Source: CAD feature listing. Evaluate the final solid. Frame: model axes, mm. A direction names the side the tool comes from. Round coordinates to 2 decimals unless told otherwise and drop trailing zeros. Order: outer loops, then holes, each group sorted by start corner. A loop starts at its lowest first (then second) coordinate and runs counter-clockwise, first axis right, second up. Notation, with made-up numbers: (79.25, 20) - (103.25, 20) arc R29 ccw to (103.25, 52) - close; hole circle Ø3 at (79, -39.75). An arc over 180 degrees is marked (long way). Put each result on its own line as item: value. Start each with the question number.
1) Section C-C on z = 39.5. Output: boundary loops of the cut face in (x, y), then the cut area to 3 significant figures.
2) Section D-D on y = 13. State how many separate pieces and enclosed holes the cut face has, then the cut area to 3 significant figures.
3) Mould query, pull axis Z, two halves, no side actions, for faces 1 (the face through (-17, 3, 30)), 2 (the face through (-23, 8, -15.011)), 3 (the face through (7, 16, 29)), 4 (the face through (-52.111, 9.409, 60.233)). Classes: +Z half, -Z half, draft (parallel to the pull), parting line (faces both ways), or undercut.
4) Section A-A on x = -7. Output: boundary loops of the cut face in (y, z).
5) Section B-B on z = 29. Output: boundary loops of the cut face in (x, y), then the cut area to 3 significant figures.
6) Line query: probe 1 along X at (y, z) = (14.5, 50); probe 2 along Z at (x, y) = (-12.5, 8.75); probe 3 along X at (y, z) = (11.25, 65.5). Output: solid intervals per line, ascending. Write a range as [from, to].
7) Contact query for flat-ended pins moving along their axis: P1, Ø1, axis at y = 8.5, z = 35, coming from the -X side; P2, Ø14.5, axis at x = -33.5, z = 29, coming from the +Y side; P3, Ø1.5, axis at x = -51, z = 66.5, coming from the +Y side. Output: stop coordinate, or through.
8) Access query for faces 5 (the face through (-57, 4, 20.989)), 6 (the face through (3.67, 10.93, 67.62)), 7 (the face through (-58.032, 11, 29)). Directions: +Z, -Z, +X, -X, +Y, -Y. A direction counts if a zero-diameter tool reaches every point of the face in a straight line with its end or side. Return the directions, or none.
Autodesk Inventor part; units mm, degrees
ref_plane "YZ Plane" through (0, 0, 0) normal (1, 0, 0) x (0, 1, 0)
ref_plane "XZ Plane" through (0, 0, 0) normal (0, 1, 0) x (-1, 0, 0)
ref_plane "XY Plane" through (0, 0, 0) normal (0, 0, 1) x (1, 0, 0)
sketch "Sketch1" plane through (0, 0, 0) normal (0, 1, 0) x (-1, 0, 0)
  line L0 (58.0321, 73.1889) -> (-11.1179, 73.1889)
  line L1 (-11.1179, 73.1889) -> (-11.1179, -15.0111)
  line L2 (-11.1179, -15.0111) -> (58.0321, -15.0111)
  line L3 (58.0321, -15.0111) -> (58.0321, 73.1889)
  point P0 (0, 0)
  dimension "d0" = 88.2
  dimension "d1" = 69.15
extrude "Extrusion1" add sketch "Sketch1" along normal blind 3
sketch "Sketch2" plane through (0, 3, 0) normal (0, 1, 0) x (1, 0, 0)
  line L0 (-58.0321, -73.1889) -> (11.1179, -73.1889)
  line L1 (11.1179, -73.1889) -> (11.1179, 15.0111)
  line L2 (-58.0321, -73.1889) -> (11.1179, -73.1889)
  line L3 (11.1179, -73.1889) -> (11.1179, 15.0111)
  line L4 (11.1179, 15.0111) -> (-58.0321, 15.0111)
  line L5 (-58.0321, 15.0111) -> (-58.0321, -73.1889)
  line L6 (-53.0321, -68.1889) -> (6.1179, -68.1889)
  line L7 (6.1179, -68.1889) -> (6.1179, 10.0111)
  line L8 (6.1179, 10.0111) -> (-53.0321, 10.0111)
  line L9 (-53.0321, 10.0111) -> (-53.0321, -68.1889)
  line L10 (-58.0321, 15.0111) -> (-58.0321, -73.1889)
  line L11 (-58.0321, -73.1889) -> (-47.0321, -73.1889)
  line L12 (-47.0321, -73.1889) -> (-47.0321, -62.1889)
  line L13 (-47.0321, -62.1889) -> (-58.0321, -62.1889)
  line L14 (-58.0321, -62.1889) -> (-58.0321, -73.1889)
  line L15 (-58.0321, 15.0111) -> (-47.0321, 15.0111)
  line L16 (-47.0321, 15.0111) -> (-47.0321, 4.0111)
  line L17 (-47.0321, 4.0111) -> (-58.0321, 4.0111)
  line L18 (-58.0321, 4.0111) -> (-58.0321, 15.0111)
  line L19 (11.1179, 15.0111) -> (0.1179, 15.0111)
  line L20 (0.1179, 15.0111) -> (0.1179, 4.0111)
  line L21 (0.1179, 4.0111) -> (11.1179, 4.0111)
  line L22 (11.1179, 4.0111) -> (11.1179, 15.0111)
  line L23 (11.1179, -73.1889) -> (0.1179, -73.1889)
  line L24 (0.1179, -73.1889) -> (0.1179, -62.1889)
  line L25 (0.1179, -62.1889) -> (11.1179, -62.1889)
  line L26 (11.1179, -62.1889) -> (11.1179, -73.1889)
  arc A0 (1.3427, -62.1889) -> (6.1179, -57.4137) centre (1.3427, -57.4137) ccw
  arc A1 (-4.6573, -68.1889) -> (0.1179, -63.4137) centre (-4.6573, -63.4137) ccw
  arc A2 (-47.0321, -63.4137) -> (-42.2569, -68.1889) centre (-42.2569, -63.4137) ccw
  arc A3 (-53.0321, -57.4137) -> (-48.2569, -62.1889) centre (-48.2569, -57.4137) ccw
  arc A4 (-48.2569, 4.0111) -> (-53.0321, -0.7641) centre (-48.2569, -0.7641) ccw
  arc A5 (-42.2569, 10.0111) -> (-47.0321, 5.2359) centre (-42.2569, 5.2359) ccw
  arc A6 (0.1179, 5.2359) -> (-4.6573, 10.0111) centre (-4.6573, 5.2359) ccw
  arc A7 (6.1179, -0.7641) -> (1.3427, 4.0111) centre (1.3427, -0.7641) ccw
  point P0 (0, 0)
  dimension "d4" = 5
  dimension "d5" = 5
  dimension "d6" = 5
  dimension "d7" = 5
  dimension "d8" = 6
  dimension "d9" = 6
  dimension "d10" = 6
  dimension "d11" = 6
  dimension "d12" = 6
  dimension "d13" = 6
  dimension "d14" = 6
  dimension "d15" = 6
  dimension "d16" = 4.7752
  dimension "d17" = 4.7752
  dimension "d18" = 4.7752
  dimension "d19" = 4.7752
  dimension "d20" = 4.7752
  dimension "d21" = 4.7752
  dimension "d22" = 4.7752
  dimension "d23" = 4.7752
  dimension "d24" = 4.7752
  dimension "d25" = 4.7752
  dimension "d26" = 4.7752
  dimension "d27" = 4.7752
  dimension "d28" = 4.7752
  dimension "d29" = 4.7752
  dimension "d30" = 4.7752
  dimension "d31" = 4.7752
  dimension "d32" = 4.7752
  dimension "d33" = 4.7752
  dimension "d34" = 4.7752
  dimension "d35" = 4.7752
  dimension "d36" = 4.7752
  dimension "d37" = 4.7752
  dimension "d38" = 4.7752
  dimension "d39" = 4.7752
extrude "Extrusion3" add sketch "Sketch2" along normal blind 13 contours L5 L13 L9 L6 L12 L0 | L12 L6 L24 L0 | L5 L17 L9 L13 | L24 L6 L7 L25 L1 L0 | L12 A2 L6 | L6 L9 L13 L12 | L5 L4 L16 L8 L9 L17 | L9 A3 L13 | L24 L25 L7 L6 | L6 A1 L24 | L17 A4 L9 | L9 L8 L16 L17 | L25 L7 L21 L1 | L4 L20 L8 L16 | L21 L7 L8 L20 L4 L1 | L25 A0 L7 | L8 A5 L16 | L21 L20 L8 L7 | L7 A7 L21 | L20 A6 L8
fillet "Fillet1" radius 4.7752 4 edges at (0.1179, 9.5, 62.1889) (-47.0321, 9.5, 62.1889) (-47.0321, 9.5, -4.0111) (0.1179, 9.5, -4.0111)
fillet "Fillet2" radius 10 4 edges at (11.1179, 8, 73.1889) (-58.0321, 8, 73.1889) (11.1179, 8, -15.0111) (-58.0321, 8, -15.0111)
sketch "Sketch4" plane through (11.1179, 0, 63.1889) normal (1, 0, 0) x (0, 0, -1)
  point P0 (63.1889, 0)
sketch "Sketch5" plane through (-58.0321, 0, -5.0111) normal (-1, 0, 0) x (0, 0, 1)
  line L0 (68.2, 0) -> (0, 0)
  line L1 (42.2, 0) -> (26, 0)
  line L2 (26, 0) -> (26, 10)
  line L3 (26, 10) -> (42.2, 10)
  line L4 (42.2, 10) -> (42.2, 0)
  line L5 (78.2, 0) -> (78.2, 16)
  line L6 (-10, 16) -> (-10, 0)
  arc A0 (42.2, 8.73) -> (40.93, 10) centre (40.5854, 8.3854) ccw
  arc A1 (27.27, 10) -> (26, 8.73) centre (27.6146, 8.3854) ccw
  point P0 (5.0111, 0)
  dimension "d48" = 10
  dimension "d49" = 16.2
  dimension "d50" = 1.27
  dimension "d51" = 1.27
  dimension "d52" = 1.27
  dimension "d53" = 1.27
  dimension "d54" = 1.651
  dimension "d55" = 1.651
  dimension "d58" = 88.2
  dimension "d59" = 36
  dimension "d60" = 36
extrude "Extrusion4" cut sketch "Sketch5" against normal blind 3 contours L0 L2 A1 L3 A0 L4
sketch "Sketch7" plane through (0, 16, 0) normal (0, 1, 0) x (1, 0, 0)
  line L0 (-53.0321, -0.7641) -> (-53.0321, -57.4137)
  line L1 (-53.0321, -43.5889) -> (-55.0321, -43.5889)
  line L2 (-55.0321, -43.5889) -> (-55.0321, -14.5889)
  line L3 (-55.0321, -14.5889) -> (-53.0321, -14.5889)
  line L4 (-53.0321, -14.5889) -> (-53.0321, -43.5889)
  line L5 (-48.0321, -73.1889) -> (1.1179, -73.1889)
  line L6 (1.1179, 15.0111) -> (-48.0321, 15.0111)
  line L7 (-55.0321, -43.5889) -> (-20.0321, -43.5889)
  line L8 (-20.0321, -43.5889) -> (-20.0321, -14.5889)
  line L9 (-20.0321, -14.5889) -> (-55.0321, -14.5889)
  line L10 (-55.0321, -14.5889) -> (-55.0321, -43.5889)
  arc A0 (-55.0321, -38.5089) -> (-49.9521, -43.5889) centre (-50.2673, -38.8241) ccw
  arc A1 (-49.9521, -14.5889) -> (-55.0321, -19.6689) centre (-50.2673, -19.3536) ccw
  arc A2 (-25.1121, -43.5889) -> (-20.0321, -38.5089) centre (-24.7969, -38.8241) ccw
  arc A3 (-20.0321, -19.6689) -> (-25.1121, -14.5889) centre (-24.7969, -19.3536) ccw
  point P0 (0, 0)
  dimension "d61" = 29.6
  dimension "d62" = 88.2
  dimension "d63" = 29
  dimension "d64" = 2
  dimension "d65" = 35
  dimension "d66" = 5.08
  dimension "d67" = 5.08
  dimension "d68" = 5.08
  dimension "d69" = 5.08
  dimension "d70" = 5.08
  dimension "d71" = 5.08
  dimension "d72" = 5.08
  dimension "d73" = 5.08
  dimension "d75" = 4.7752
  dimension "d76" = 4.7752
  dimension "d77" = 4.7752
  dimension "d78" = 29
  dimension "d82" = 4.7752
  dimension "d107" = 18.84
extrude "Extrusion5" cut sketch "Sketch7" against normal blind 14 contours A1 L9 A3 L8 A2 L7 A0 L0 | L0 A0 L2 A1 | A1 L9 | L2 A1 | A0 L2 | L7 A0 | A3 L9 | L7 A2 | A3 L8 | L8 A2
fillet "Fillet3" radius 4.7752 2 edges at (-53.0321, 9.5, 42.7175) (-53.0321, 9.5, 15.4602)
sketch "Sketch8" plane through (0, 16, 0) normal (0, 1, 0) x (1, 0, 0)
  line L0 (-48.0321, -73.1889) -> (1.1179, -73.1889)
  line L1 (-58.0321, 5.0111) -> (-58.0321, -63.1889)
  line L2 (11.1179, -63.1889) -> (11.1179, 5.0111)
  line L3 (1.1179, 15.0111) -> (-48.0321, 15.0111)
  point P0 (0, 0)
  point P1 (-51.0321, 8.0111)
  point P2 (4.1179, 8.0111)
  point P3 (4.1179, -66.1889)
  point P4 (-51.0321, -66.1889)
  dimension "d83" = 7
  dimension "d84" = 7
  dimension "d85" = 7
  dimension "d86" = 7
  dimension "d87" = 7
  dimension "d88" = 7
  dimension "d89" = 7
  dimension "d90" = 7
hole "Hole1" at (-51.0321, 16, -8.0111) at (4.1179, 16, -8.0111) at (4.1179, 16, 66.1889) at (-51.0321, 16, 66.1889) direction (0, -1, 0) diameter 3 depth 10
sketch "Sketch9" plane through (0, 3, 0) normal (0, 1, 0) x (1, 0, 0)
  line L0 (1.1179, 15.0111) -> (-48.0321, 15.0111)
  line L1 (-58.0321, 5.0111) -> (-58.0321, -63.1889)
  point P0 (0, 0)
  point P1 (-40.2521, -5.3089)
  dimension "d98" = 20.32
  dimension "d99" = 17.78
hole "Hole2" at (-40.2521, 3, 5.3089) direction (0, -1, 0) diameter 3.75 depth 10
equation "\"d5\" = d4"
equation "\"d6\" = d4"
equation "\"d7\" = d4"
equation "\"d9\" = d8"
equation "\"d10\" = d8"
equation "\"d11\" = d8"
equation "\"d12\" = d8"
equation "\"d14\" = d8"
equation "\"d15\" = d9"
equation "\"d17\" = d16"
equation "\"d18\" = d16"
equation "\"d19\" = d18"
equation "\"d25\" = d24"
equation "\"d26\" = d25"
equation "\"d27\" = d25"
equation "\"d28\" = d21"
equation "\"d29\" = d28"
equation "\"d30\" = d16"
equation "\"d31\" = d28"
equation "\"d32\" = d31"
equation "\"d33\" = d30"
equation "\"d34\" = d31"
equation "\"d35\" = d34"
equation "\"d36\" = d33"
equation "\"d37\" = d34"
equation "\"d38\" = d37"
equation "\"d39\" = d36"
equation "\"d51\" = d50"
equation "\"d52\" = d50"
equation "\"d53\" = d50"
equation "\"d54\" = d55"
equation "\"d59\" = -0.5 * d49 + 0.5 * d58"
equation "\"d61\" = -0.5 * d63 + 0.5 * d62"
equation "\"d67\" = d66"
equation "\"d68\" = d67"
equation "\"d69\" = d68"
equation "\"d70\" = d67"
equation "\"d71\" = d70"
equation "\"d72\" = d73"
equation "\"d73\" = d71"
equation "\"d76\" = d74"
equation "\"d77\" = d74"
equation "\"d78\" = d63"
equation "\"d82\" = d75"
properties part number "macropad-frame-v2"
Answer sheet:
1. outline: (-58.03, 0) - (11.12, 0) - (11.12, 16) - (6.12, 16) - (6.12, 3) - (-20.07, 3) - (-20.07, 2) - (-54.99, 2) - (-54.99, 16) - (-58.03, 16) - close
1. area: 277 mm^2
2. separate pieces: 1
2. enclosed holes: 5
2. area: 1,480 mm^2
3. face 1: undercut
3. face 2: -Z half
3. face 3: draft
3. face 4: undercut
4. outline: (0, -15.01) - (16, -15.01) - (16, -10.01) - (3, -10.01) - (3, 68.19) - (16, 68.19) - (16, 73.19) - (0, 73.19) - close
5. outline: (-58.03, 10) - (-55.03, 10) - (-55.03, 16) - (-58.03, 16) - close; (-55.03, 0) - (11.12, 0) - (11.12, 16) - (6.12, 16) - (6.12, 3) - (-20.03, 3) - (-20.03, 2) - (-55.03, 2) - close
5. area: 246 mm^2
6. probe 1: [-58.03, -53.03], [6.12, 11.12]
6. probe 2: [-15.01, -10.01], [68.19, 73.19]
6. probe 3: [-57.76, -52.36], [-49.7, -46.55], [-0.36, 2.79], [5.45, 10.85]
7. P1: x = 6.12
7. P2: y = 2
7. P3: y = 6
8. face 5: -X, -Y
8. face 6: +Y
8. face 7: +Z, -Z, -X, +Y, -Y
